Verification items for the finished model (mm, model axes). A direction names the side the tool comes from. Coordinates: 2 decimals unless noted, no trailing zeros. Order: outer loops, then holes, each group sorted by start corner. A loop starts at its lowest first (then second) coordinate and runs counter-clockwise, first axis right, second up. Notation, with made-up numbers: (-2, 22) -> (14, 22) arc R13 ccw to (14, 46) -> close; hole circle Ø7 at (51.25, -14.5). An arc over 180 degrees is marked (long way). Answer as CSV lines item,"result".
```python
from build123d import *

# Parameters (mm, degrees)
BOSS_EXTRUDE1_DEPTH      = 12.7
SKETCH2_R                = 1.5875
SIDE_MOUNT_HOLES_DEPTH   = 6.35
SKETCH3_R                = 1.5875
BOTTOM_MOUNT_HOLES_DEPTH = 3.81
FILLET1_R                = 6.35
FILLET2_R                = 2.54
SKETCH4_R                = 2.159
SWITCH_MOUNT_HOLES_DEPTH = 7.112
SKETCH5_R                = 2.159
CUT_EXTRUDE1_DEPTH       = 7.112
FILLET3_R                = 1.27


with BuildPart() as part:
    # Sketch1 → Boss-Extrude1 (new body)
    with BuildSketch(Plane.XY):
        Polygon((19.05, 0), (-19.05, 0), (-19.05, 3.81), (-6.35, 3.81), (-6.35, 105.41), (-97.4598, 105.41), (-97.4598, 92.71), (-101.2698, 92.71), (-101.2698, 130.81), (-97.4598, 130.81), (-97.4598, 118.11), (97.4598, 118.11), (97.4598, 130.81), (101.2698, 130.81), (101.2698, 92.71), (97.4598, 92.71), (97.4598, 105.41), (6.35, 105.41), (6.35, 3.81), (19.05, 3.81), align=None)
    extrude(amount=BOSS_EXTRUDE1_DEPTH)

    # Sketch2 → Side-Mount-Holes (cut)
    with BuildSketch(Plane(origin=(101.2698, 0, 0), x_dir=(0, 0, -1), z_dir=(1, 0, 0))):
        with Locations(Location((-6.35, 124.46, 0), (0, 0, 90))):
            Circle(SKETCH2_R)
        with Locations(Location((-6.35, 99.06, 0), (0, 0, 90))):
            Circle(SKETCH2_R)
    side_mount_holes = extrude(amount=-SIDE_MOUNT_HOLES_DEPTH, mode=Mode.SUBTRACT)

    # Mirror1: Side-Mount-Holes across plane
    add(side_mount_holes.mirror(Plane(origin=(0, 0, 0), x_dir=(0, 0, 1), z_dir=(1, 0, 0))), mode=Mode.SUBTRACT)

    # Sketch3 → Bottom_Mount_Holes (cut)
    with BuildSketch(Plane.XZ):
        with Locations((12.7, 6.35)):
            Circle(SKETCH3_R)
        with Locations(Location((-12.7, 6.35, 0), (0, 0, 270))):
            Circle(SKETCH3_R)
    extrude(amount=-BOTTOM_MOUNT_HOLES_DEPTH, mode=Mode.SUBTRACT)

    # Fillet1
    fillet1_edges = [part.edges().sort_by_distance(p)[0] for p in [
        (-6.35, 105.41, 6.35),
        (6.35, 105.41, 6.35),
    ]]
    fillet(fillet1_edges, radius=FILLET1_R)

    # Fillet2
    fillet2_edges = [part.edges().sort_by_distance(p)[0] for p in [
        (-6.35, 3.81, 6.35),
        (-97.4598, 105.41, 6.35),
        (-97.4598, 118.11, 6.35),
        (97.4598, 118.11, 6.35),
        (97.4598, 105.41, 6.35),
        (6.35, 3.81, 6.35),
    ]]
    fillet(fillet2_edges, radius=FILLET2_R)

    # Sketch4 → Switch_Mount_Holes (cut)
    with BuildSketch(Plane(origin=(6.35, 0, 0), x_dir=(0, 0, -1), z_dir=(1, 0, 0))):
        with Locations(Location((-6.35, 53.975, 0), (0, 0, 90))):
            Circle(SKETCH4_R)
        with Locations(Location((-6.35, 34.925, 0), (0, 0, 270))):
            Circle(SKETCH4_R)
    extrude(amount=-SWITCH_MOUNT_HOLES_DEPTH, mode=Mode.SUBTRACT)

    # Sketch5 → Cut-Extrude1 (cut)
    with BuildSketch(Plane(origin=(0, 118.11, 0), x_dir=(1, 0, 0), z_dir=(0, 1, 0))):
        with Locations(Location((-12.7, -6.35, 0), (0, 0, 180))):
            Circle(SKETCH5_R)
        with Locations((12.7, -6.35)):
            Circle(SKETCH5_R)
    extrude(amount=-CUT_EXTRUDE1_DEPTH, mode=Mode.SUBTRACT)

    # Fillet3
    fillet3_edges = [part.edges().sort_by_distance(p)[0] for p in [
        (-19.05, 3.81, 6.35),
        (-97.4598, 92.71, 6.35),
        (-101.2698, 92.71, 6.35),
        (-101.2698, 130.81, 6.35),
        (-97.4598, 130.81, 6.35),
        (97.4598, 130.81, 6.35),
        (101.2698, 130.81, 6.35),
        (101.2698, 92.71, 6.35),
        (97.4598, 92.71, 6.35),
        (19.05, 3.81, 6.35),
        (19.05, 0, 6.35),
        (-19.05, 0, 6.35),
    ]]
    fillet(fillet3_edges, radius=FILLET3_R)


solid = part.part
```
Item 1: Depth check by flat-ended pin: pin 1 Ø12 at (x, y) = (7, 28.5) entering from +Z; pin 2 Ø4 at (y, z) = (58.5, 7.5) entering from -X; pin 3 Ø2 at (x, z) = (1, 9) entering from +Y; pin 4 Ø2.5 at (y, z) = (53.975, 6.35) entering from +X. Enter the tip coordinate at first touch or a pass-through.
Answer list:
pin 1,"z = 12.7"
pin 2,"x = -6.35"
pin 3,"y = 118.11"
pin 4,"x = -0.76"
Item 2: Release check for a two-part mould opening along Y. For faces 6 (the flat face through (97.46, 97, 6)), 7 (the flat face through (-13, 110.998, 6)), 8 (the cylindrical face through (8.26, 103.6, 6.44)) record: +Y half, -Y half, draft (parallel to the pull), parting line (faces both ways), or undercut.
Answer list:
face 6,"draft"
face 7,"+Y half"
face 8,"undercut"
Item 3: Thickness scan on line 1 (Z direction, x = -99.2, y = 124.46); line 2 (X direction, y = 104.5, z = 3.25); line 3 (Y direction, x = 50, z = 11.75). Record the ranges inside material, lowest first.
Answer list:
line 1,"0 to 4.76, 7.94 to 12.7"
line 2,"-101.27 to -96.87, -9.42 to 9.42, 96.87 to 101.27"
line 3,"105.41 to 118.11"
Item 4: Section check B-B, the plane x = -56.5. Record the boundary of the cut face in (y, z), plus the area to 3 significant figures.
Answer list:
outline,"(105.41, 0) -> (118.11, 0) -> (118.11, 12.7) -> (105.41, 12.7) -> close"
area,"161 mm2"
Item 5: Section check A-A, the plane y = 61. Record the boundary of the cut face in (x, z).
Answer list:
outline,"(-6.35, 0) -> (6.35, 0) -> (6.35, 12.7) -> (-6.35, 12.7) -> close"
Item 6: Tool access check on faces 1 (the flat face through (-14, 3.81, 5)), 2 (the flat face through (-1, 118.11, 6)), 3 (the cylindrical face through (2.84, 35.39, 8.46)), 4 (the flat face through (13, 110.998, 6)), 5 (the flat face through (-97.46, 97, 5)). Record the directions out of +Z, -Z, +X, -X, +Y, -Y that give a thin tool (end or side, any length) a straight path to the whole face; none if there is none.
Answer list:
face 1,"+Z, -Z, -X"
face 2,"+Z, -Z, +Y"
face 3,"+X"
face 4,"+Y"
face 5,"+Z, -Z, -Y"
